Work out the finished part from the listing and answer in its coordinate system (mm). A direction names the side the tool comes from. Round coordinates to 2 decimals unless told otherwise and drop trailing zeros. Loops run counter-clockwise (first coordinate to the right, second up) from the corner with the lowest first, then second, coordinate; pieces in that order, holes last.
```python
from build123d import *

# Parameters (mm, degrees)
SKETCH1_R           = 16.637
BOSS_EXTRUDE1_DEPTH = 21.844
SKETCH2_W           = 25.4
SKETCH2_H           = 6.35
BOSS_EXTRUDE2_DEPTH = 24.003
SKETCH3_W           = 25.4
SKETCH3_H           = 6.35
BOSS_EXTRUDE3_DEPTH = 24.003
SKETCH4_R           = 4.7625
CUT_EXTRUDE1_DEPTH  = 20.812
FILLET1_R           = 3.175


with BuildPart() as part:
    # Sketch1 → Boss-Extrude1 (new body)
    with BuildSketch(Plane.XY):
        Circle(SKETCH1_R)
    extrude(amount=BOSS_EXTRUDE1_DEPTH)

    # Sketch2 → Boss-Extrude2 (add)
    with BuildSketch(Plane.XY.offset(21.844)):
        Rectangle(SKETCH2_W, SKETCH2_H)
    extrude(amount=BOSS_EXTRUDE2_DEPTH)

    # Sketch3 → Boss-Extrude3 (add)
    with BuildSketch(Plane(origin=(0, 0, 0), x_dir=(-1, 0, 0), z_dir=(0, 0, -1))):
        Rectangle(SKETCH3_W, SKETCH3_H)
    extrude(amount=BOSS_EXTRUDE3_DEPTH)

    # Sketch4 → Cut-Extrude1 (cut, through all)
    with BuildSketch(Plane(origin=(0, 3.175, 0), x_dir=(1, 0, 0), z_dir=(0, 1, 0))):
        with Locations((0, 12.446)):
            Circle(SKETCH4_R)
        with Locations((0, -34.29)):
            Circle(SKETCH4_R)
    extrude(amount=-CUT_EXTRUDE1_DEPTH, mode=Mode.SUBTRACT)

    # Fillet1
    fillet1_edges = [part.edges().sort_by_distance(p)[0] for p in [
        (-16.637, 0, 0),
        (-16.637, 0, 21.844),
    ]]
    fillet(fillet1_edges, radius=FILLET1_R)


solid = part.part
```
1. Consider probe 1 along Z at (x, y) = (0, 1); probe 2 along X at (y, z) = (2, 34); probe 3 along Z at (x, y) = (-3, 1.5). Determine where each line is inside the solid, lowest interval first.
Answer key:
probe 1: z = -24 to -17.21, -7.68 to 29.53, 39.05 to 45.85
probe 2: x = -12.7 to -4.75, 4.75 to 12.7
probe 3: z = -24 to -16.14, -8.75 to 30.59, 37.99 to 45.85
2. Find section B-B (x = 0). Give the number of separate pieces and of enclosed holes in the cut face, then the cut area to 3 significant figures.
Answer key:
separate pieces: 3
enclosed holes: 0
area: 902 mm2
3. Which of the six approach directions +Z, -Z, +X, -X, +Y, -Y give full straight-line access (tool end or side, diameter ignored) to faces 5 (the face through (12.7, 0, -12)), 6 (the face through (0, -3.175, 28)), 7 (the face through (0, 3.175, -6)), 8 (the face through (-12.7, 0, -12))?
Answer key:
face 5: -Z, +X, +Y, -Y
face 6: +Z, +X, -X, -Y
face 7: -Z, +X, -X, +Y
face 8: -Z, -X, +Y, -Y
4. Given pin 1 (6 mm diameter, centred on x = -7.5, z = 18.5, fed in from +Y); pin 2 (3 mm diameter, centred on y = 1, z = -11.5, fed in from +X); pin 3 (5 mm diameter, centred on x = 9, z = 26.5, fed in from +Y) (3 decimals), each flat-ended and moving along its own axis, determine where each tip first touches the part or whether it passes through.
Answer key:
pin 1: stops at y = 16.02
pin 2: stops at x = 12.7
pin 3: stops at y = 3.175
5. Determine the mould class of faces 1 (the face through (0, -3.175, -6)), 2 (the face through (-0.62, 0.044, -17.168)), 3 (the face through (0, 0, -24.003)), 4 (the face through (-0.62, 0.04, 29.57)) for opening direction Z: +Z half, -Z half, draft (parallel to the pull), parting line (faces both ways), or undercut.
Answer key:
face 1: draft
face 2: undercut
face 3: -Z half
face 4: undercut
6. Find section A-A (z = 34.29). Write down the section's boundary in (x, y) (1 decimal).
Answer key:
outline: (-12.7, -3.2) - (-4.8, -3.2) - (-4.8, 3.2) - (-12.7, 3.2) - close; (4.8, -3.2) - (12.7, -3.2) - (12.7, 3.2) - (4.8, 3.2) - close
7. Find section D-D (z = -14). Write down the section's boundary in (x, y) (3 decimals).
Answer key:
outline: (-12.7, -3.175) - (-4.502, -3.175) - (-4.502, 3.175) - (-12.7, 3.175) - close; (4.502, -3.175) - (12.7, -3.175) - (12.7, 3.175) - (4.502, 3.175) - close
